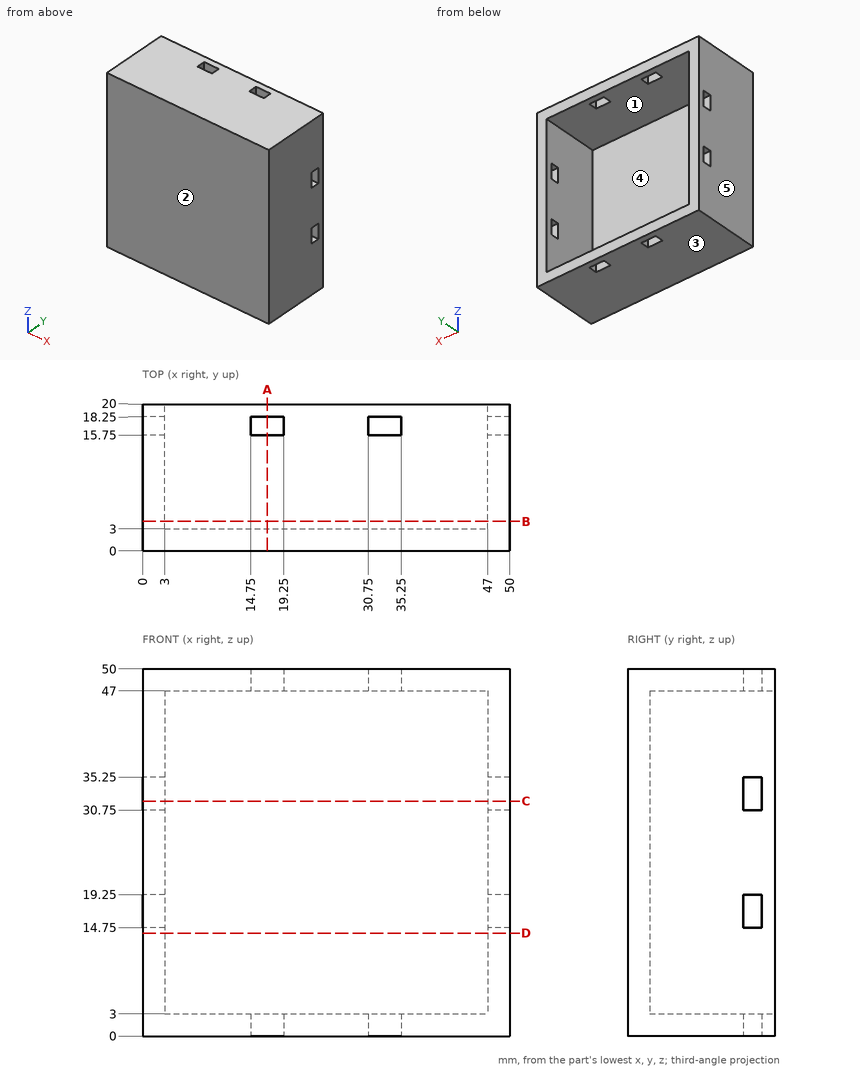
Check sheet for the drawn part. Datum: minimum x, y, z corner. Units: mm. A direction names the side the tool comes from. Give positions to 0.01 mm unless a question says otherwise; leave off trailing zeros. Write each loop counter-clockwise with the first axis right and the second up, starting at its lowest first coordinate (ties: lowest second). Pieces come first, ordered by that corner, then holes. Notation, with made-up numbers: M 85.5,-35 L 100.5,-35 A9 cw 100.5,-22 Z; hole C 84.5,20 d9. An arc over 180 degrees is marked long. One line per question, with ' | ' between items.
1) Thickness scan on line 1 along Z through (x, y) = (12, 7.5); line 2 along Z through (x, y) = (48.5, 17.25). Record the ranges inside material, lowest first. Write a range as [from, to].
Result:
line 1: z = [0, 3], [47, 50] | line 2: z = [0, 14.75], [19.25, 30.75], [35.25, 50]
2) Mould release check, pull along Z, two halves, no side actions. Record for the marked faces 1, 2 and 3: released by +Z, released by -Z, zero draft, split by the parting line, or undercut.
Result:
face 1: undercut | face 2: zero draft | face 3: released by -Z
3) Section check C-C on z = 32. Enter the section's corners in (x, y).
Result:
outline: M 0,0 L 50,0 L 50,15.75 L 47,15.75 L 47,3 L 3,3 L 3,15.75 L 0,15.75 Z; M 0,18.25 L 3,18.25 L 3,20 L 0,20 Z; M 47,18.25 L 50,18.25 L 50,20 L 47,20 Z
4) Section check A-A on x = 17. Enter the section's corners in (y, z), plus the area to 3 significant figures.
Result:
outline: M 0,0 L 15.75,0 L 15.75,3 L 3,3 L 3,47 L 15.75,47 L 15.75,50 L 0,50 Z; M 18.25,0 L 20,0 L 20,3 L 18.25,3 Z; M 18.25,47 L 20,47 L 20,50 L 18.25,50 Z | area: 237 mm2
5) Section check D-D on z = 14. Enter the section's corners in (x, y), plus the area to 3 significant figures.
Result:
outline: M 0,0 L 50,0 L 50,20 L 47,20 L 47,3 L 3,3 L 3,20 L 0,20 Z | area: 252 mm2
6) Section check B-B on y = 4. Enter the section's corners in (x, z), plus the area to 3 significant figures.
Result:
outline: M 0,0 L 50,0 L 50,50 L 0,50 Z; hole M 3,3 L 47,3 L 47,47 L 3,47 Z | area: 564 mm2
7) Set-up check for the marked faces 4 and 5: record each of +Z, -Z, +X, -X, +Y, -Y from which the full face is reachable in a straight line by a thin tool's end or side.
Result:
face 4: +Y | face 5: +Z, -Z, -X, +Y, -Y
